```python
from build123d import *

# Parameters (mm, degrees)
F0_R      = 3
F1_DEPTH  = 3
F2_W      = 10
F2_H      = 3
F2_W_2    = 14
F3_DEPTH  = 10
F5_DEPTH  = 3
F6_R      = 4.8
F6_R_2    = 2.5
F7_DEPTH  = 2
F9_DEPTH  = 25
F10_R     = 5
F11_R     = 1.5
F12_DEPTH = 25


with BuildPart() as f1:
    # F0 (on Top) → F1 (new body)
    with BuildSketch(Plane.XY):
        with BuildLine():
            Line((0, 0), (3, 0))
            Line((3, 0), (97, 0))
            Line((97, 0), (100, 0))
            Line((100, 0), (100, 33))
            Line((100, 33), (96, 33))
            ThreePointArc((96, 33), (94, 35), (96, 37))
            Line((96, 37), (100, 37))
            Line((100, 37), (100, 63.000004))
            Line((100, 63.000004), (96.003777, 63.000004))
            ThreePointArc((96.003777, 63.000004), (94.000001, 64.998112), (96, 67))
            Line((96, 67), (100, 67))
            Line((100, 67), (100, 102))
            Line((100, 102), (97, 102))
            Line((97, 102), (3, 102))
            Line((3, 102), (0, 102))
            Line((0, 102), (0, 0))
        make_face()
        with Locations((38, 50)):
            Circle(F0_R, mode=Mode.SUBTRACT)
        with BuildLine():
            Line((10, 14), (10, 35))
            ThreePointArc((10, 35), (10.87868, 37.12132), (13, 38))
            Line((13, 38), (14.296335, 38))
            Line((14.296335, 38), (14.296335, 42))
            ThreePointArc((14.296335, 42), (15.175015, 44.12132), (17.296335, 45))
            Line((17.296335, 45), (26, 45))
            Line((26, 45), (29, 45))
            ThreePointArc((29, 45), (29.169876, 45.004813), (29.339751, 45))
            ThreePointArc((29.339751, 45), (30.972651, 44.402729), (32, 43))
            Line((32, 43), (52, 43))
            ThreePointArc((52, 43), (53.166024, 44.500964), (55, 45))
            Line((55, 45), (73.5, 45))
            ThreePointArc((73.5, 45), (75.62132, 44.12132), (76.5, 42))
            Line((76.5, 42), (76.5, 40))
            Line((76.5, 40), (87, 40))
            ThreePointArc((87, 40), (89.12132, 39.12132), (90, 37))
            Line((90, 37), (90, 35.75))
            Line((90, 35.75), (90, 16.5))
            Line((90, 16.5), (90, 8))
            ThreePointArc((90, 8), (89.12132, 5.87868), (87, 5))
            Line((87, 5), (82, 5))
            ThreePointArc((82, 5), (81.414214, 3.585786), (80, 3))
            Line((80, 3), (70, 3))
            ThreePointArc((70, 3), (68.585786, 3.585786), (68, 5))
            Line((68, 5), (55, 5))
            ThreePointArc((55, 5), (52.87868, 5.87868), (52, 8))
            Line((52, 8), (32, 8))
            ThreePointArc((32, 8), (31.12132, 5.87868), (29, 5))
            Line((29, 5), (24, 5))
            Line((24, 5), (18, 5))
            ThreePointArc((18, 5), (15.87868, 5.87868), (15, 8))
            Line((15, 8), (15, 11))
            Line((15, 11), (13, 11))
            ThreePointArc((13, 11), (10.87868, 11.87868), (10, 14))
        make_face(mode=Mode.SUBTRACT)
        with BuildLine():
            Line((16, 97), (26, 97))
            Line((26, 97), (52, 97))
            Line((52, 97), (52, 98))
            ThreePointArc((52, 98), (52.87868, 100.12132), (55, 101))
            Line((55, 101), (62, 101))
            ThreePointArc((62, 101), (64.12132, 100.12132), (65, 98))
            Line((65, 98), (65, 97))
            Line((65, 97), (74, 97))
            ThreePointArc((74, 97), (76.12132, 96.12132), (77, 94))
            Line((77, 94), (77, 88.5))
            Line((77, 88.5), (77, 82.5))
            Line((77, 82.5), (83, 82.5))
            ThreePointArc((83, 82.5), (85.12132, 81.62132), (86, 79.5))
            Line((86, 79.5), (86, 67))
            Line((86, 67), (89, 67))
            ThreePointArc((89, 67), (91.12132, 66.12132), (92, 64))
            Line((92, 64), (92, 60))
            ThreePointArc((92, 60), (91.12132, 57.87868), (89, 57))
            Line((89, 57), (72, 57))
            ThreePointArc((72, 57), (70.585786, 57.585786), (70, 59))
            Line((70, 59), (30, 59))
            ThreePointArc((30, 59), (29.414214, 57.585786), (28, 57))
            Line((28, 57), (23, 57))
            Line((23, 57), (16, 57))
            ThreePointArc((16, 57), (13.87868, 57.87868), (13, 60))
            ThreePointArc((13, 60), (10.87868, 60.87868), (10, 63))
            Line((10, 63), (10, 91))
            ThreePointArc((10, 91), (10.87868, 93.12132), (13, 94))
            ThreePointArc((13, 94), (13.87868, 96.12132), (16, 97))
        make_face(mode=Mode.SUBTRACT)
    extrude(amount=F1_DEPTH)

    # F2 (on face) → F3 (join)
    with BuildSketch(Plane.XY.offset(3)):
        with Locations((5, 26.5)):
            Rectangle(F2_W, F2_H)
        with Locations((95, 26.5)):
            Rectangle(F2_W, F2_H)
        with Locations((5, 74.5)):
            Rectangle(F2_W, F2_H)
        with Locations((93, 74.5)):
            Rectangle(F2_W_2, F2_H)
    extrude(amount=F3_DEPTH)

    # F4 (on face) → F5 (join)
    with BuildSketch(Plane.XY.offset(13)):
        with BuildLine():
            Line((0, 28), (0, 25))
            Line((0, 25), (33.675445, 25))
            ThreePointArc((33.675445, 25), (40, 20), (46.324555, 25))
            Line((46.324555, 25), (100, 25))
            Line((100, 25), (100, 28))
            Line((100, 28), (46.324555, 28))
            ThreePointArc((46.324555, 28), (40, 33), (33.675445, 28))
            Line((33.675445, 28), (0, 28))
        make_face()
        with BuildLine():
            Line((100, 73), (100, 76))
            Line((100, 76), (39.324555, 76))
            ThreePointArc((39.324555, 76), (33, 81), (26.675445, 76))
            Line((26.675445, 76), (0, 76))
            Line((0, 76), (0, 73))
            Line((0, 73), (26.675445, 73))
            ThreePointArc((26.675445, 73), (33, 68), (39.324555, 73))
            Line((39.324555, 73), (100, 73))
        make_face()
    extrude(amount=F5_DEPTH)

    # F6 (on face) → F7 (cut)
    with BuildSketch(Plane(origin=(0, 0, 13), x_dir=(1, 0, 0), z_dir=(0, 0, -1))):
        with Locations((40, -26.5)):
            Circle(F6_R)
        with Locations((40, -26.5)):
            Circle(F6_R_2, mode=Mode.SUBTRACT)
        with Locations((33, -74.5)):
            Circle(F6_R)
        with Locations((33, -74.5)):
            Circle(F6_R_2, mode=Mode.SUBTRACT)
    extrude(amount=-F7_DEPTH, mode=Mode.SUBTRACT)

    # F8 (on face) → F9 (cut)
    with BuildSketch(Plane.XY.offset(3)):
        with BuildLine():
            Line((93, 54), (49, 54))
            ThreePointArc((49, 54), (46.87868, 53.12132), (46, 51))
            ThreePointArc((46, 51), (46.87868, 48.87868), (49, 48))
            Line((49, 48), (93, 48))
            ThreePointArc((93, 48), (95.12132, 48.87868), (96, 51))
            ThreePointArc((96, 51), (95.12132, 53.12132), (93, 54))
        make_face()
        with BuildLine():
            ThreePointArc((90, 80), (90.87868, 77.87868), (93, 77))
            Line((93, 77), (94, 77))
            ThreePointArc((94, 77), (96.12132, 77.87868), (97, 80))
            Line((97, 80), (97, 92))
            ThreePointArc((97, 92), (96.12132, 94.12132), (94, 95))
            Line((94, 95), (93, 95))
            ThreePointArc((93, 95), (90.87868, 94.12132), (90, 92))
            Line((90, 92), (90, 80))
        make_face()
        with BuildLine():
            Line((2, 22), (2, 9))
            ThreePointArc((2, 9), (2.87868, 6.87868), (5, 6))
            ThreePointArc((5, 6), (7.12132, 6.87868), (8, 9))
            Line((8, 9), (8, 22))
            ThreePointArc((8, 22), (7.12132, 24.12132), (5, 25))
            ThreePointArc((5, 25), (2.87868, 24.12132), (2, 22))
        make_face()
        with BuildLine():
            ThreePointArc((31, 51), (30.12132, 53.12132), (28, 54))
            Line((28, 54), (6, 54))
            ThreePointArc((6, 54), (3.87868, 53.12132), (3, 51))
            ThreePointArc((3, 51), (3.87868, 48.87868), (6, 48))
            Line((6, 48), (28, 48))
            ThreePointArc((28, 48), (30.12132, 48.87868), (31, 51))
        make_face()
    extrude(amount=-F9_DEPTH, mode=Mode.SUBTRACT)

    # F10
    f10_edges = [f1.edges().sort_by_distance(p)[0] for p in [
        (33.675445, 25, 14.5),
        (46.324555, 25, 14.5),
        (46.324555, 28, 14.5),
        (39.324555, 76, 14.5),
        (33.675445, 28, 14.5),
        (26.675445, 76, 14.5),
        (26.675445, 73, 14.5),
        (39.324555, 73, 14.5),
    ]]
    fillet(f10_edges, radius=F10_R)

    # F11 (on face) → F12 (cut)
    with BuildSketch(Plane(origin=(0, 0, 13), x_dir=(1, 0, 0), z_dir=(0, 0, -1))):
        with Locations((40, -26.5)):
            Circle(F11_R)
        with Locations((33, -74.5)):
            Circle(F11_R)
    extrude(amount=-F12_DEPTH, mode=Mode.SUBTRACT)


solid = f1.part
```
CAD build for the part. Positions are in the model's coordinates, mm. A direction names the side the tool comes from. Give positions to 0.01 mm unless a question says otherwise; leave off trailing zeros. Order: outer loops, then holes, each group sorted by start corner. A loop starts at its lowest first (then second) coordinate and runs counter-clockwise, first axis right, second up. Notation, with made-up numbers: M -24,66.5 L 18,66.5 A10 ccw 18,70.5 Z; hole C 37.25,1 d2. An arc over 180 degrees is marked long. Put each result on its own line as item: value. Start each with the question number.
(1) Saw through at D-D, the plane y = 18. Write the cut outline in (x, z).
(2) Saw through at A-A, the plane y = 85.5. Write the cut outline in (x, z).
(3) Which spindle directions (+Z, -Z, +X, -X, +Y, -Y) get a long thin tool onto all of the face, cutting with end or side? Do faces 1 (the flat face through (90, 23.6, 2.6)), 2 (the cylindrical face through (47.13, 28.59, 14.52)), 3 (the cylindrical face through (13.86, 96.1, 1.48)). Say none if no direction does.
(4) Saw through at B-B, the plane x = 21. Write the cut outline in (y, z), then the cut area to 3 significant figures.
(5) Flat gauge pins, fed straight in: pin 1 Ø5 at (y, z) = (68, 13) entering from -X; pin 2 Ø7.5 at (x, y) = (40, 26.5) entering from -Z; pin 3 Ø12 at (x, y) = (51, 89) entering from +Z. Where does each tip first touch, or does it go through?
(6) Saw through at C-C, the plane y = 74.5. Write the cut outline in (x, z), then the cut area to 3 significant figures.
(7) Mould opens along Y. For faces 4 (the flat face through (100, 50, 1)), 5 (the cylindrical face through (38.89, 25.49, 14.48)), 6 (the cylindrical face through (31.14, 5.9, 1.48)) say: +Y half, -Y half, draft (parallel to the pull), parting line (faces both ways), or undercut.
(8) Drill centre lines: line 1 along X through (y, z) = (74.5, 14.2); line 2 along X through (y, z) = (87, 2); line 3 along Y through (x, z) = (40, 13.95). Where is each one in solid material? Low to high.
Check result:
1. outline: M 0,0 L 2,0 L 2,3 L 0,3 Z; M 8,0 L 10,0 L 10,3 L 8,3 Z; M 90,0 L 100,0 L 100,3 L 90,3 Z
2. outline: M 0,0 L 10,0 L 10,3 L 0,3 Z; M 77,0 L 90,0 L 90,3 L 77,3 Z; M 97,0 L 100,0 L 100,3 L 97,3 Z
3. face 1: -Z
3. face 2: +Z, -Z, +X
3. face 3: +Z, -Z
4. outline: M 0,0 L 5,0 L 5,3 L 0,3 Z; M 25,13 L 28,13 L 28,16 L 25,16 Z; M 45,0 L 48,0 L 48,3 L 45,3 Z; M 54,0 L 57,0 L 57,3 L 54,3 Z; M 73,13 L 76,13 L 76,16 L 73,16 Z; M 97,0 L 102,0 L 102,3 L 97,3 Z
4. area: 66.0 mm2
5. pin 1: stops at x = 27.88
5. pin 2: stops at z = 13
5. pin 3: passes through
6. outline: M 0,0 L 10,0 L 10,13 L 28.2,13 L 28.2,15 L 30.5,15 L 30.5,13 L 31.5,13 L 31.5,16 L 0,16 Z; M 34.5,13 L 35.5,13 L 35.5,15 L 37.8,15 L 37.8,13 L 86,13 L 86,0 L 100,0 L 100,16 L 34.5,16 Z
6. area: 594 mm2
7. face 4: draft
7. face 5: undercut
7. face 6: undercut
8. line 1: x = 0 to 28.2, 30.5 to 31.5, 34.5 to 35.5, 37.8 to 100
8. line 2: x = 0 to 10, 77 to 90, 97 to 100
8. line 3: y = 20 to 21.7, 24 to 25, 28 to 29, 31.3 to 33, 72.34 to 76.66
